Geometry: final body of the model. Coordinates: model frame, mm. A direction names the side the tool comes from. Coordinates: 2 decimals unless noted, no trailing zeros. Loops run counter-clockwise (first coordinate to the right, second up) from the corner with the lowest first, then second, coordinate; pieces in that order, holes last. Notation, with made-up numbers: (49, 46.25) - (59, 46.25) arc R29 ccw to (59, 70.25) - close; hole circle Ø9 at (-39, 43). An arc over 180 degrees is marked (long way). Put each result on its own line as item: value. Start each with the question number.
1) Section C-C on y = 13.25. Output: boundary loops of the cut face in (x, z), and give its area (3 significant figures).
2) Material intervals for line 1 along X through (y, z) = (1.75, 0); line 2 along X through (y, z) = (12.25, 0); line 3 along X through (y, z) = (23, -7), sorted ascending. Write a range as from..to.
3) Section D-D on x = -54.5. Output: boundary loops of the cut face in (y, z).
4) Section B-B on x = 60. Output: boundary loops of the cut face in (y, z).
5) Draft query along X for faces 4 (the cylindrical face through (-62.351, 15.325, 1.223)), 5 (the flat face through (62, 28, -2)), 6 (the flat face through (75, 11, 1)). Return one class per face: +X half, -X half, draft (parallel to the pull), parting line (faces both ways), or undercut.
6) Reachability of faces 1 (the flat face through (-63, 15, 10)), 2 (the flat face through (-50, 15, 0)), 3 (the flat face through (-62, 15, -10)) from +Z, -Z, +X, -X, +Y, -Y: full face, straight path, thin tool, end or side. Return the list, or none.
7) Section A-A on z = 0. Output: boundary loops of the cut face in (x, y).
8) Contact query for flat-ended pins moving along their axis: pin 1 Ø1.6 at (x, z) = (-60, 0.5) entering from +Y; pin 2 Ø3 at (x, z) = (-56, -31) entering from +Y; pin 3 Ø12.5 at (x, y) = (-63.5, 12.5) entering from -Z. Output: stop coordinate, or through.
```python
from build123d import *

# Parameters (mm, degrees)
SKETCH1_W           = 150
SKETCH1_H           = 100
SKETCH1_R           = 2.6
BOSS_EXTRUDE1_DEPTH = 3
SKETCH2_R           = 2.65
BOSS_EXTRUDE2_DEPTH = 25
FILLET1_R           = 10


with BuildPart() as part:
    # Sketch1 → Boss-Extrude1 (new body)
    with BuildSketch(Plane(origin=(0, 0, 0), x_dir=(1, 0, 0), z_dir=(0, 1, 0))):
        Rectangle(SKETCH1_W, SKETCH1_H)
        with Locations(Location((-60, 0, 0), (0, 0, 270))):
            Circle(SKETCH1_R, mode=Mode.SUBTRACT)
        with Locations(Location((60, 0, 0), (0, 0, 270))):
            Circle(SKETCH1_R, mode=Mode.SUBTRACT)
    extrude(amount=BOSS_EXTRUDE1_DEPTH)

    # Sketch2 → Boss-Extrude2 (add)
    # profile 1 of 2: a face of its own
    with BuildSketch(Plane(origin=(0, 3, 0), x_dir=(1, 0, 0), z_dir=(0, 1, 0))):
        Polygon((-70, -10), (-50, -10), (-50, 10), (-70, 10), (-75, 10), (-75, -10), align=None)
        with Locations(Location((-60, 0, 0), (0, 0, 270))):
            Circle(SKETCH2_R, mode=Mode.SUBTRACT)
    # profile 2 of 2: a face of its own
    with BuildSketch(Plane(origin=(0, 3, 0), x_dir=(1, 0, 0), z_dir=(0, 1, 0))):
        Polygon((49.997605223, -10.002394777), (70.002394777, -10.002394777), (75, -10.002394777), (75, 10.002394777), (70.002394777, 10.002394777), (49.997605223, 10.002394777), align=None)
        with Locations(Location((60, 0, 0), (0, 0, 270))):
            Circle(SKETCH2_R, mode=Mode.SUBTRACT)
    extrude(amount=BOSS_EXTRUDE2_DEPTH)

    # Fillet1
    fillet1_edges = [part.edges().sort_by_distance(p)[0] for p in [
        (75, 1.5, 50),
        (-75, 1.5, 50),
        (-75, 1.5, -50),
        (75, 1.5, -50),
    ]]
    fillet(fillet1_edges, radius=FILLET1_R)


solid = part.part
```
Answer block:
1. outline: (-75, -10) - (-50, -10) - (-50, 10) - (-75, 10) - close; (50, -10) - (75, -10) - (75, 10) - (50, 10) - close; hole circle Ø5.3 at (-60, 0); hole circle Ø5.3 at (60, 0)
1. area: 956 mm²
2. line 1: x = -75..-62.6, -57.4..57.4, 62.6..75
2. line 2: x = -75..-62.65, -57.35..-50, 50..57.35, 62.65..75
2. line 3: x = -75..-50, 50..75
3. outline: (0, -50) - (3, -50) - (3, -10) - (28, -10) - (28, 10) - (3, 10) - (3, 50) - (0, 50) - close
4. outline: (0, -50) - (3, -50) - (3, -10) - (28, -10) - (28, -2.65) - (3, -2.65) - (3, -2.6) - (0, -2.6) - close; (0, 2.6) - (3, 2.6) - (3, 2.65) - (28, 2.65) - (28, 10) - (3, 10) - (3, 50) - (0, 50) - close
5. face 4: undercut
5. face 5: draft
5. face 6: +X half
6. face 1: +Z, +X, -X, +Y
6. face 2: +Z, -Z, +Y
6. face 3: -Z, +X, -X, +Y
7. outline: (-75, 0) - (-62.6, 0) - (-62.6, 3) - (-62.65, 3) - (-62.65, 28) - (-75, 28) - close; (-57.4, 0) - (57.4, 0) - (57.4, 3) - (57.35, 3) - (57.35, 28) - (50, 28) - (50, 3) - (-50, 3) - (-50, 28) - (-57.35, 28) - (-57.35, 3) - (-57.4, 3) - close; (62.6, 0) - (75, 0) - (75, 28) - (62.65, 28) - (62.65, 3) - (62.6, 3) - close
8. pin 1: passes through
8. pin 2: stops at y = 3
8. pin 3: stops at z = -10
